Can you work these out from the drawing? Everything is in mm from the part's minimum corner. Coordinates: 2 decimals unless noted, no trailing zeros. Loops run counter-clockwise (first coordinate to the right, second up) from the corner with the lowest first, then second, coordinate; pieces in that order, holes last. Notation, with made-up numbers: (88.25, -18.75) -> (135.25, -18.75) arc R15 ccw to (135.25, -4.75) -> close; hole circle Ø9 at (64, 25). An arc over 180 degrees is marked (long way). Use one line per item in the form item = value. Start each with the question number.
(1) Imagine slicing it at B-B (z = 27.94). List the corners of the cut face in (x, y) for me, plus the area to 3 significant figures.
(2) Imagine slicing it at C-C (y = 0.2). List the corners of the cut face in (x, z) for me, plus the area to 3 significant figures.
(3) Imagine slicing it at A-A (x = 8.89). List the corners of the cut face in (y, z) for me.
(4) I need wall thicknesses on line 1 (Z direction, x = 8.89, y = 0.5); line 2 (X direction, y = 0.6, z = 2.5); line 3 (X direction, y = 0.15, z = 29). Which ranges of each line are inside material? Lowest first, please. Write a range as [from, to].
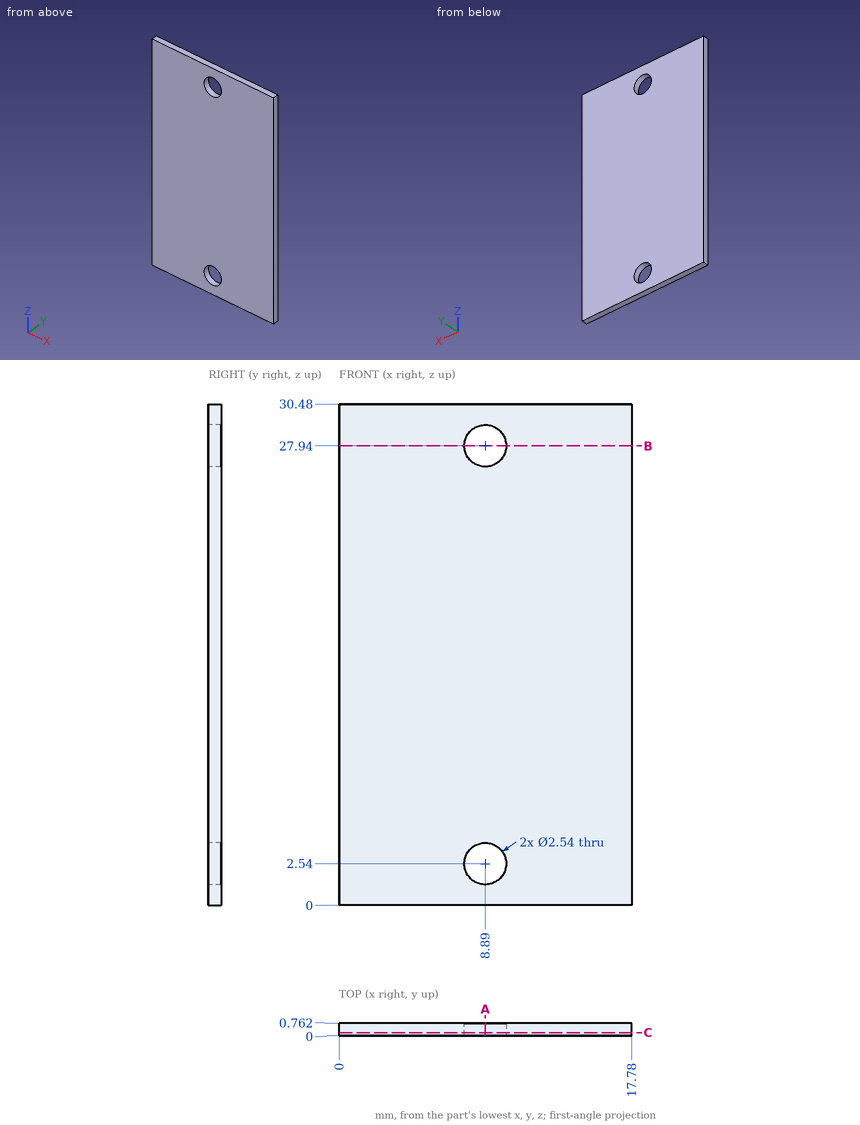
Worked out:
q1.outline = (0, 0) -> (7.62, 0) -> (7.62, 0.76) -> (0, 0.76) -> close; (10.16, 0) -> (17.78, 0) -> (17.78, 0.76) -> (10.16, 0.76) -> close
q1.area = 11.6 mm2
q2.outline = (0, 0) -> (17.78, 0) -> (17.78, 30.48) -> (0, 30.48) -> close; hole circle Ø2.54 at (8.89, 2.54); hole circle Ø2.54 at (8.89, 27.94)
q2.area = 532 mm2
q3.outline = (0, 0) -> (0.76, 0) -> (0.76, 1.27) -> (0, 1.27) -> close; (0, 3.81) -> (0.76, 3.81) -> (0.76, 26.67) -> (0, 26.67) -> close; (0, 29.21) -> (0.76, 29.21) -> (0.76, 30.48) -> (0, 30.48) -> close
q4.line_1 = [0, 1.27], [3.81, 26.67], [29.21, 30.48]
q4.line_2 = [0, 7.62], [10.16, 17.78]
q4.line_3 = [0, 8.19], [9.59, 17.78]
